Build history of the part. All positions in model axes, mm. A direction names the side the tool comes from. Round coordinates to 2 decimals unless told otherwise and drop trailing zeros. Write each loop counter-clockwise with the first axis right and the second up, starting at its lowest first coordinate (ties: lowest second). Pieces come first, ordered by that corner, then holes. Notation, with made-up numbers: (41.25, 27.5) - (86.25, 27.5) arc R22 cw to (86.25, 37.5) - close; hole circle Ø7 at (14.5, 12). An arc over 180 degrees is marked (long way). Answer as a JSON object with one key per item and string values. Group by question number.
Item 1: Slice it at A-A, the plane z = 33. List the corners of the cut face in (x, y).
Item 2: Slice it at B-B, the plane x = 0. List the corners of the cut face in (y, z).
Item 3: Which spindle directions (+Z, -Z, +X, -X, +Y, -Y) get a long thin tool onto all of the face, cutting with end or side? Do faces 1 (the cylindrical face through (-41.1, -0.53, 2.94)), 2 (the flat face through (42.91, -25.22, 35.15)). Say none if no direction does.
Item 4: Slice it at D-D, the plane x = -25.4. List the corners of the cut face in (y, z), then the cut area to 3 significant figures.
Item 5: Flat gauge pins, fed straight in: pin 1 (3 mm diameter, centred on x = 8, y = -6.5, fed in from -Z); pin 2 (6 mm diameter, centred on x = -8.5, y = -17.5, fed in from +Z); pin 3 (4.5 mm diameter, centred on x = 0, y = 25.4, fed in from +Z). Where does each tip first touch, or does it go through?
Item 6: Probe line 1 (Y direction, x = 0, z = 0.55); line 2 (Y direction, x = -25, z = 1); line 3 (Y direction, x = 25.4, z = 1.65). List the from-to ranges inside material, lowest first. Write a range as from..to.
Item 7: Slice it at C-C, the plane y = 0. Give the number of separate pieces and of enclosed holes in the cut face, then the cut area to 3 significant figures.
Item 8: Two-plate mould, pull along Y, no slides. Class faces 3 (the flat face through (-42.94, -25.22, 35.15)), 4 (the cylindrical face through (0.46, 21.86, 1.16)), 5 (the cylindrical face through (-42.765, -0.533, 1.375)): +Y half, -Y half, draft (parallel to the pull), parting line (faces both ways), or undercut.
from build123d import *

# Parameters (mm, degrees)
F1_DEPTH = 38.1
F2_R     = 4.7625
F3_DEPTH = 88.139
F5_D     = 7.1374


with BuildPart() as f1:
    # F0 (on Front) → F1 (new body, symmetric)
    with BuildSketch(Plane.XZ):
        with BuildLine():
            Line((44.069, 4.572), (44.069, 50.8))
            Line((44.069, 50.8), (41.783, 50.8))
            Line((41.783, 50.8), (41.783, 4.572))
            ThreePointArc((41.783, 4.572), (41.113446, 2.955554), (39.497, 2.286))
            Line((39.497, 2.286), (-39.497, 2.286))
            ThreePointArc((-39.497, 2.286), (-41.113446, 2.955554), (-41.783, 4.572))
            Line((-41.783, 4.572), (-41.783, 50.8))
            Line((-41.783, 50.8), (-44.069, 50.8))
            Line((-44.069, 50.8), (-44.069, 4.572))
            ThreePointArc((-44.069, 4.572), (-42.729892, 1.339108), (-39.497, 0))
            Line((-39.497, 0), (39.497, 0))
            ThreePointArc((39.497, 0), (42.729892, 1.339108), (44.069, 4.572))
        make_face()
    extrude(amount=F1_DEPTH, both=True)

    # F2 (on face) → F3 (cut, through all)
    with BuildSketch(Plane(origin=(-44.069, 0, 0), x_dir=(0, -1, 0), z_dir=(-1, 0, 0))):
        Polygon((12.7, 50.8), (38.1, 19.05), (38.1, 50.8), align=None)
        with Locations((0, 44.789256)):
            Circle(F2_R)
        Polygon((-38.1, 19.05), (-12.7, 50.8), (-38.1, 50.8), align=None)
    extrude(amount=-F3_DEPTH, mode=Mode.SUBTRACT)

    # F5 (through all)
    with Locations(Plane(origin=(0, 0, 0), x_dir=(1, 0, 0), z_dir=(0, 0, -1))):
        with Locations((0, 25.4), (25.4, 0), (0, 0), (-25.4, 0), (-25.4, -25.4), (0, -25.4), (25.4, -25.4)):
            Hole(F5_D / 2)


solid = f1.part
Geometry says:
{
 "1": {"outline": "(-44.07, -26.94) - (-41.78, -26.94) - (-41.78, 26.94) - (-44.07, 26.94) - close; (41.78, -26.94) - (44.07, -26.94) - (44.07, 26.94) - (41.78, 26.94) - close"},
 "2": {"outline": "(-38.1, 0) - (-28.97, 0) - (-28.97, 2.29) - (-38.1, 2.29) - close; (-21.83, 0) - (-3.57, 0) - (-3.57, 2.29) - (-21.83, 2.29) - close; (3.57, 0) - (21.83, 0) - (21.83, 2.29) - (3.57, 2.29) - close; (28.97, 0) - (38.1, 0) - (38.1, 2.29) - (28.97, 2.29) - close"},
 "3": {"face 1": "+Z, +Y, -Y", "face 2": "+Z, +X, -X, -Y"},
 "4": {"outline": "(-38.1, 0) - (-3.57, 0) - (-3.57, 2.29) - (-38.1, 2.29) - close; (3.57, 0) - (21.83, 0) - (21.83, 2.29) - (3.57, 2.29) - close; (28.97, 0) - (38.1, 0) - (38.1, 2.29) - (28.97, 2.29) - close", "area": "142 mm^2"},
 "5": {"pin 1": "stops at z = 0", "pin 2": "stops at z = 2.29", "pin 3": "passes through"},
 "6": {"line 1": "y = -38.1..-28.97, -21.83..-3.57, 3.57..21.83, 28.97..38.1", "line 2": "y = -38.1..-3.55, 3.55..21.85, 28.95..38.1", "line 3": "y = -38.1..-3.57, 3.57..21.83, 28.97..38.1"},
 "7": {"separate pieces": "6", "enclosed holes": "0", "area": "324 mm^2"},
 "8": {"face 3": "-Y half", "face 4": "undercut", "face 5": "draft"}
}
